Read the model definition and answer for the solid it produces. Units are mm, in the model's axes. A direction names the side the tool comes from. Give positions to 0.01 mm unless a question says otherwise; leave off trailing zeros. Write each loop counter-clockwise with the first axis right and the second up, starting at its lowest first coordinate (ties: lowest second). Pieces come first, ordered by that corner, then holes.
```python
from build123d import *

# Parameters (mm, degrees)
SKETCH1_R           = 2.5
BOSS_EXTRUDE1_DEPTH = 5
SKETCH2_W           = 10
SKETCH2_H           = 10
BOSS_EXTRUDE2_DEPTH = 5


with BuildPart() as part:
    # Sketch1 → Boss-Extrude1 (new body)
    with BuildSketch(Plane.XY):
        with BuildLine():
            ThreePointArc((5, 0), (-3.535533906, 3.535533906), (0, -5))
            Line((0, -5), (20, -5))
            ThreePointArc((20, -5), (23.535533906, 3.535533906), (15, 0))
            Line((15, 0), (5, 0))
        make_face()
        with Locations((20, 0)):
            Circle(SKETCH1_R, mode=Mode.SUBTRACT)
        Circle(SKETCH1_R, mode=Mode.SUBTRACT)
    extrude(amount=BOSS_EXTRUDE1_DEPTH)

    # Sketch2 → Boss-Extrude2 (add)
    with BuildSketch(Plane(origin=(0, 0, 0), x_dir=(1, 0, 0), z_dir=(0, 1, 0))):
        with Locations((10, -2.5)):
            Rectangle(SKETCH2_W, SKETCH2_H)
    extrude(amount=-BOSS_EXTRUDE2_DEPTH)


solid = part.part
```
Item 1: Determine the mould class of faces 6 (the flat face through (2, -2, 5)), 7 (the cylindrical face through (17.5, 0.1, 2.5)), 8 (the cylindrical face through (-0.54, -2.44, 2.46)), 9 (the flat face through (15, -2, -1)) for opening direction X: pulls with the +X half, pulls with the -X half, needs draft (parallel to the pull), parting line crosses it, or undercut.
Result set:
face 6: needs draft
face 7: undercut
face 8: undercut
face 9: pulls with the +X half
Item 2: Section B-B (x = 1.5) is taken. Write down the section's boundary in (y, z), and give its area (3 significant figures).
Result set:
outline: (-5, 0) - (-2, 0) - (-2, 5) - (-5, 5) - close; (2, 0) - (4.77, 0) - (4.77, 5) - (2, 5) - close
area: 28.8 mm2
Item 3: Section A-A (y = -3) is taken. Write down the section's boundary in (x, z), and give its area (3 significant figures).
Result set:
outline: (-4, 0) - (5, 0) - (5, -2.5) - (15, -2.5) - (15, 0) - (24, 0) - (24, 5) - (15, 5) - (15, 7.5) - (5, 7.5) - (5, 5) - (-4, 5) - close
area: 190 mm2
Item 4: Find the intervals of material crossed by line 1 along Y through (x, z) = (20, 1.9); line 2 along X through (y, z) = (2.25, 2.75); line 3 along Z through (x, y) = (-1.5, -4), in increasing order.
Result set:
line 1: y = -5 to -2.5, 2.5 to 5
line 2: x = -4.47 to -1.09, 1.09 to 4.47, 15.53 to 18.91, 21.09 to 24.47
line 3: z = 0 to 5
Item 5: Each of these flat-tipped pins is pushed along its axis until it touches: pin 1 Ø0.8 at (y, z) = (-2.5, -1) entering from -X; pin 2 Ø3 at (x, y) = (18, -2) entering from +Z; pin 3 Ø5 at (x, y) = (-1.5, 0.5) entering from -Z. Where does it stop, or does it pass through?
Result set:
pin 1: stops at x = 5
pin 2: stops at z = 5
pin 3: stops at z = 0
Item 6: Section D-D (y = 3.5) is taken. Write down the section's boundary in (x, z).
Result set:
outline: (-3.57, 0) - (3.57, 0) - (3.57, 5) - (-3.57, 5) - close; (16.43, 0) - (23.57, 0) - (23.57, 5) - (16.43, 5) - close
Item 7: Which of the six approach directions +Z, -Z, +X, -X, +Y, -Y give full straight-line access (tool end or side, diameter ignored) to faces 1 (the flat face through (18, -2, 0)), 2 (the flat face through (10, 0, 2)), 3 (the flat face through (18, -2, 5)), 4 (the flat face through (5, -2, 6)), 5 (the flat face through (2, -2, 0))?
Result set:
face 1: -Z, +X, +Y, -Y
face 2: +Z, -Z, +Y
face 3: +Z, +X, +Y, -Y
face 4: +Z, -X, +Y, -Y
face 5: -Z, -X, +Y, -Y
Item 8: Section C-C (z = 1.5) is taken. Write down the section's boundary in (x, y).
Result set:
outline: (0, -5) - (20, -5) arc R5 ccw (long way) to (15, 0) - (5, 0) arc R5 ccw (long way) to start; hole circle Ø5 at (0, 0); hole circle Ø5 at (20, 0)
